from build123d import *

# Parameters (mm, degrees)
SKETCH_2_W          = 30
SKETCH_2_H          = 20
EXTRUDE_1_DEPTH     = 3
FILLET_1_R          = 3
SKETCH_3_R          = 1.6
CUT_EXTRUDE_1_DEPTH = 4
EXTRUDE_2_DEPTH     = 3
FILLET_2_R          = 1


with BuildPart() as part:
    # 草图2 → 凸台-拉伸1 (new body)
    with BuildSketch(Plane.XY):
        with Locations((15, -10)):
            Rectangle(SKETCH_2_W, SKETCH_2_H)
    extrude(amount=EXTRUDE_1_DEPTH)

    # 圆角1
    fillet_1_edges = [part.edges().sort_by_distance(p)[0] for p in [
        (0, 0, 1.5),
        (30, 0, 1.5),
        (30, -20, 1.5),
        (0, -20, 1.5),
    ]]
    fillet(fillet_1_edges, radius=FILLET_1_R)

    # 草图3 → 切除-拉伸1 (cut, through all)
    with BuildSketch(Plane.XY.offset(3)):
        with Locations((23, -2.5)):
            Circle(SKETCH_3_R)
        with Locations((23, -17.5)):
            Circle(SKETCH_3_R)
        with Locations((7, -17.5)):
            Circle(SKETCH_3_R)
        with Locations((7, -2.5)):
            Circle(SKETCH_3_R)
    extrude(amount=-CUT_EXTRUDE_1_DEPTH, mode=Mode.SUBTRACT)

    # 草图4 → 凸台-拉伸2 (add)
    with BuildSketch(Plane(origin=(0, 0, 0), x_dir=(-1, 0, 0), z_dir=(0, 0, -1))):
        Polygon((0, -10), (0, -13), (3, -13), (3, -7), (0, -7), align=None)
    extrude(amount=-EXTRUDE_2_DEPTH)

    # 圆角2
    fillet_2_edges = [part.edges().sort_by_distance(p)[0] for p in [
        (0, -7, 1.5),
        (-3, -7, 1.5),
        (-3, -13, 1.5),
        (0, -13, 1.5),
    ]]
    fillet(fillet_2_edges, radius=FILLET_2_R)


solid = part.part
Design review of the part built by this model. Coordinates are the model's own, in mm. A direction names the side the tool comes from. Give positions to 0.01 mm unless a question says otherwise; leave off trailing zeros. Loops run counter-clockwise (first coordinate to the right, second up) from the corner with the lowest first, then second, coordinate; pieces in that order, holes last. Notation, with made-up numbers: M -24.5,-10.75 L 12.5,-10.75 A21 ccw 12.5,0.25 Z; hole C 23,70.5 d9. An arc over 180 degrees is marked long. Answer as a JSON object with one key per item and string values.
Item 1: Wall thickness on line 1 along Y through (x, z) = (7, 1.35); line 2 along X through (y, z) = (-3.5, 2.6); line 3 along X through (y, z) = (-6, 2): over which ranges is each line inside the solid? List them lowest first.
Output values:
{"line 1": "y = -20 to -19.1, -15.9 to -4.1, -0.9 to 0", "line 2": "x = 0 to 5.75, 8.25 to 21.75, 24.25 to 30", "line 3": "x = 0 to 30"}
Item 2: We need section A-A (x = 7). State the section outline as (y, z) points.
Output values:
{"outline": "M -20,0 L -19.1,0 L -19.1,3 L -20,3 Z; M -15.9,0 L -4.1,0 L -4.1,3 L -15.9,3 Z; M -0.9,0 L 0,0 L 0,3 L -0.9,3 Z"}
Item 3: Mouldability with a two-part tool opening along Y and no side actions: class faces 1 (the face through (30, -10, 1)), 2 (the face through (6.792, -15.914, 1.521)), 3 (the face through (29.14, -0.9, 1.52)), 4 (the face through (24.526, -2.019, 1.521)) as pulls with the +Y half, pulls with the -Y half, needs draft (parallel to the pull), parting line crosses it, or undercut.
Output values:
{"face 1": "needs draft", "face 2": "undercut", "face 3": "pulls with the +Y half", "face 4": "undercut"}
Item 4: Machinability: for faces 5 (the face through (13, -10, 0)), 6 (the face through (-1.5, -13, 1.5)), 7 (the face through (-1.5, -7, 1.5)), which of the approach directions +Z, -Z, +X, -X, +Y, -Y give a long, thin tool a straight path to every point of the face, cutting with its end or side? Answer none if there is none.
Output values:
{"face 5": "-Z, +X, -X, +Y, -Y", "face 6": "+Z, -Z, -X, -Y", "face 7": "+Z, -Z, -X, +Y"}
Item 5: We need section D-D (y = -13.5). State the section outline as (x, z) points.
Output values:
{"outline": "M -0.13,0 L 30,0 L 30,3 L -0.13,3 Z"}
Item 6: We need section B-B (z = 1.8). State the section outline as (x, y) points.
Output values:
{"outline": "M -3,-12 A1 ccw -2,-13 L -1,-13 A1 cw 0,-14 L 0,-17 A3 ccw 3,-20 L 27,-20 A3 ccw 30,-17 L 30,-3 A3 ccw 27,0 L 3,0 A3 ccw 0,-3 L 0,-6 A1 cw -1,-7 L -2,-7 A1 ccw -3,-8 Z; hole C 7,-17.5 d3.2; hole C 7,-2.5 d3.2; hole C 23,-17.5 d3.2; hole C 23,-2.5 d3.2"}
Item 7: We need section C-C (y = -16.25). State the section outline as (x, z) points.
Output values:
{"outline": "M 0,0 L 6,0 L 6,3 L 0,3 Z; M 8,0 L 22,0 L 22,3 L 8,3 Z; M 24,0 L 30,0 L 30,3 L 24,3 Z"}
Item 8: For P1, Ø3.5, axis at x = 7, y = -2.5, coming from the -Z side; P2, Ø1.5, axis at y = -15, z = 2, coming from the -X side; P3, Ø0.5, axis at x = -1.5, z = 1, coming from the +Y side, all flat-tipped, find the tip position at first contact; note any pin that passes through.
Output values:
{"P1": "stops at z = 0", "P2": "stops at x = 0", "P3": "stops at y = -7"}
